```python
from build123d import *

# Parameters (mm, degrees)
CROQUIS1_R              = 3.8
SALIENTE_EXTRUIR1_DEPTH = 10
CROQUIS3_R              = 10
SALIENTE_EXTRUIR2_DEPTH = 2
SALIENTE_EXTRUIR3_DEPTH = 7
CROQUIS6_R              = 6
CORTAR_EXTRUIR6_DEPTH   = 0.5


with BuildPart() as part:
    # Croquis1 → Saliente-Extruir1 (new body)
    with BuildSketch(Plane.XY):
        Circle(CROQUIS1_R)
    extrude(amount=SALIENTE_EXTRUIR1_DEPTH)

    # Croquis3 → Saliente-Extruir2 (add)
    with BuildSketch(Plane(origin=(0, 0, 0), x_dir=(-1, 0, 0), z_dir=(0, 0, -1))):
        Circle(CROQUIS3_R)
    extrude(amount=SALIENTE_EXTRUIR2_DEPTH)

    # Croquis4 → Saliente-Extruir3 (add)
    with BuildSketch(Plane(origin=(0, 0, -2), x_dir=(-1, 0, 0), z_dir=(0, 0, -1))):
        Polygon((3.75277675, -6.5), (7.505553499, 0), (3.75277675, 6.5), (-3.75277675, 6.5), (-7.505553499, 0), (-3.75277675, -6.5), align=None)
    extrude(amount=SALIENTE_EXTRUIR3_DEPTH)

    # Croquis6 → Cortar-Extruir6 (cut)
    with BuildSketch(Plane(origin=(0, 0, -9), x_dir=(-1, 0, 0), z_dir=(0, 0, -1))):
        Circle(CROQUIS6_R)
    extrude(amount=-CORTAR_EXTRUIR6_DEPTH, mode=Mode.SUBTRACT)

    # Croquis7 → Cortar-Revolución1 (revolve, cut)
    with BuildSketch(Plane(origin=(0, 0, 0), x_dir=(1, 0, 0), z_dir=(0, 1, 0))):
        Polygon((-5.5, 15.2), (-5.5, 9.932050808), (-8.5, 8.2), (-8.5, 15.2), align=None)
    revolve(axis=Axis((0, 0, 0), (0, 0, -1)), mode=Mode.SUBTRACT)


solid = part.part
```
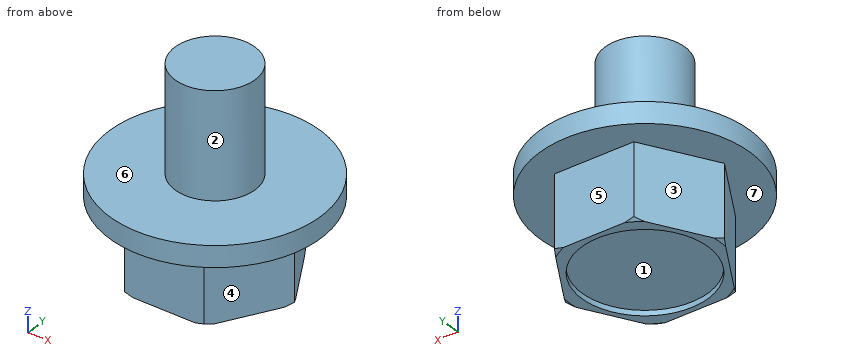
Build history of the part. All positions in model axes, mm. Face numbers are marked on the shaded views. A direction names the side the tool comes from. Give positions to 0.01 mm unless a question says otherwise; leave off trailing zeros. Loops run counter-clockwise (first coordinate to the right, second up) from the corner with the lowest first, then second, coordinate; pieces in that order, holes last.
Item 1: Drill centre lines: line 1 (Y direction, x = 0, z = -8.6); line 2 (Z direction, x = -2.5, y = 9); line 3 (Z direction, x = -2, y = 3.75). Where is each one in solid material? Low to high.
Answers follow:
line 1: y = -6.5 to -6, 6 to 6.5
line 2: z = -2 to 0
line 3: z = -8.5 to 0
Item 2: Slice it at C-C, the plane y = 3.5. List the corners of the cut face in (x, z), and give its area (3 significant figures).
Answers follow:
outline: (-9.37, -2) - (-5.48, -2) - (-5.48, -9) - (-4.87, -9) - (-4.87, -8.5) - (4.87, -8.5) - (4.87, -9) - (5.48, -9) - (5.48, -2) - (9.37, -2) - (9.37, 0) - (1.48, 0) - (1.48, 10) - (-1.48, 10) - (-1.48, 0) - (-9.37, 0) - close
area: 139 mm2
Item 3: Slice it at A-A, the plane x = 0. List the corners of the cut face in (y, z).
Answers follow:
outline: (-10, -2) - (-6.5, -2) - (-6.5, -9) - (-6, -9) - (-6, -8.5) - (6, -8.5) - (6, -9) - (6.5, -9) - (6.5, -2) - (10, -2) - (10, 0) - (3.8, 0) - (3.8, 10) - (-3.8, 10) - (-3.8, 0) - (-10, 0) - close
Item 4: Flat gauge pins, fed straight in: pin 1 (4 mm diameter, centred on x = -0.5, z = 4.5, fed in from +Y); pin 2 (3.5 mm diameter, centred on x = 2, y = -2.5, fed in from -Z); pin 3 (5 mm diameter, centred on y = -7, z = -6, fed in from -X). Where does each tip first touch, or does it go through?
Answers follow:
pin 1: stops at y = 3.8
pin 2: stops at z = -8.5
pin 3: stops at x = -4.91
Item 5: Pull direction X, two halves, no side cores. Call the marked faces 1, 2, 3 and 4: released by +X, released by -X, zero draft, split by the parting line, or undercut.
Answers follow:
face 1: undercut
face 2: split by the parting line
face 3: released by -X
face 4: released by +X
Item 6: Slice it at D-D, the plane y = 8. List the corners of the cut face in (x, z), and give its area (3 significant figures).
Answers follow:
outline: (-6, -2) - (6, -2) - (6, 0) - (-6, 0) - close
area: 24.0 mm2
Item 7: Slice it at B-B, the plane z = -3.25. List the corners of the cut face in (x, y).
Answers follow:
outline: (-7.51, 0) - (-3.75, -6.5) - (3.75, -6.5) - (7.51, 0) - (3.75, 6.5) - (-3.75, 6.5) - close
Item 8: Which spindle directions (+Z, -Z, +X, -X, +Y, -Y) get a long thin tool onto all of the face, cutting with end or side? Do the marked faces 5, 6 and 7. Say none if no direction does.
Answers follow:
face 5: -Z, +X, -X, +Y
face 6: +Z
face 7: -Z
